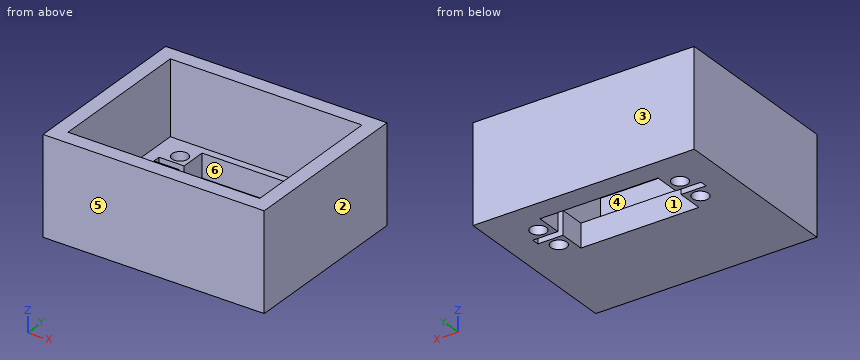
```python
from build123d import *

# Parameters (mm, degrees)
ESQUISSE1_W             = 75
ESQUISSE1_H             = 60
BOSS_EXTRU_1_DEPTH      = 8
ESQUISSE2_W             = 40
ESQUISSE2_H             = 20
ENL_V_MAT_EXTRU_1_DEPTH = 8
ESQUISSE3_W             = 8.5
ESQUISSE3_H             = 2.5
ENL_V_MAT_EXTRU_2_DEPTH = 8
ESQUISSE4_R             = 2.7
ENL_V_MAT_EXTRU_3_DEPTH = 49.685213361
ESQUISSE6_W             = 75
ESQUISSE6_H             = 60
BOSS_EXTRU_2_DEPTH      = 35
ESQUISSE7_W             = 65
ESQUISSE7_H             = 50
ENL_V_MAT_EXTRU_4_DEPTH = 35
CUT_EXTRUDE1_REACH      = 90.034
SKETCH1_W               = 10
SKETCH1_H               = 60


with BuildPart() as part:
    # Esquisse1 → Boss.-Extru.1 (new body)
    with BuildSketch(Plane.XY):
        Rectangle(ESQUISSE1_W, ESQUISSE1_H)
    extrude(amount=-BOSS_EXTRU_1_DEPTH)

    # Esquisse2 → Enlèv. mat.-Extru.1 (cut)
    with BuildSketch(Plane.XY):
        with Locations((0, 12.5)):
            Rectangle(ESQUISSE2_W, ESQUISSE2_H)
    extrude(amount=-ENL_V_MAT_EXTRU_1_DEPTH, mode=Mode.SUBTRACT)

    # Esquisse3 → Enlèv. mat.-Extru.2 (cut)
    with BuildSketch(Plane.XY):
        with Locations((-24.25, 12.5)):
            Rectangle(ESQUISSE3_W, ESQUISSE3_H)
    enl_v_mat_extru_2 = extrude(amount=-ENL_V_MAT_EXTRU_2_DEPTH, mode=Mode.SUBTRACT)

    # Esquisse4 → Enlèv. mat.-Extru.3 (cut, through all)
    with BuildSketch(Plane.XY):
        with Locations((-24, 17.5)):
            Circle(ESQUISSE4_R)
        with Locations((-24, 7.5)):
            Circle(ESQUISSE4_R)
    enl_v_mat_extru_3 = extrude(amount=-ENL_V_MAT_EXTRU_3_DEPTH, mode=Mode.SUBTRACT)

    # Symétrie2: Enlèv. mat.-Extru.2, Enlèv. mat.-Extru.3 across plane
    add(enl_v_mat_extru_2.mirror(Plane(origin=(0, 0, 0), x_dir=(0, 0, 1), z_dir=(1, 0, 0))), mode=Mode.SUBTRACT)
    add(enl_v_mat_extru_3.mirror(Plane(origin=(0, 0, 0), x_dir=(0, 0, 1), z_dir=(1, 0, 0))), mode=Mode.SUBTRACT)

    # Esquisse6 → Boss.-Extru.2 (add)
    with BuildSketch(Plane.XY):
        Rectangle(ESQUISSE6_W, ESQUISSE6_H)
    extrude(amount=BOSS_EXTRU_2_DEPTH)

    # Esquisse7 → Enlèv. mat.-Extru.4 (cut)
    with BuildSketch(Plane.XY.offset(35)):
        Rectangle(ESQUISSE7_W, ESQUISSE7_H)
    extrude(amount=-ENL_V_MAT_EXTRU_4_DEPTH, mode=Mode.SUBTRACT)

    # Cut-Extrude1: up to this face of the body (flat: up to its plane)
    cut_extrude1_end = Plane(part.part.faces().sort_by_distance((-37.5, 0, 13.5))[0])
    # Sketch1 → Cut-Extrude1 (cut, up to the picked face)
    with BuildSketch(Plane(origin=(37.5, 0, 0), x_dir=(0, 0, -1), z_dir=(1, 0, 0)), mode=Mode.PRIVATE) as cut_extrude1_sk1:
        with Locations((-30, 0)):
            Rectangle(SKETCH1_W, SKETCH1_H)
    cut_extrude1_tool1 = split(extrude(cut_extrude1_sk1.sketch, amount=-CUT_EXTRUDE1_REACH, mode=Mode.PRIVATE), bisect_by=cut_extrude1_end, keep=Keep.BOTH, mode=Mode.PRIVATE)
    add(cut_extrude1_tool1.solids().sort_by(Axis((37.5, 0, 30), (-1, 0, 0)))[0], mode=Mode.SUBTRACT)


solid = part.part
```
Part model, mm, in its own coordinate system. Face numbers are marked on the shaded views. A direction names the side the tool comes from. Round coordinates to 2 decimals unless told otherwise and drop trailing zeros. Write each loop counter-clockwise with the first axis right and the second up, starting at its lowest first coordinate (ties: lowest second). Pieces come first, ordered by that corner, then holes. Notation, with made-up numbers: M 15.25,-19.5 L 27.25,-19.5 A22 ccw 27.25,7.5 Z; hole C 79.5,-35 d8. An arc over 180 degrees is marked long. One line per question, with ' | ' between items.
(1) Probe line 1 along Y through (x, z) = (-24, -5.75); line 2 along Y through (x, z) = (-21, 23.5); line 3 along X through (y, z) = (15, 17). List the from-to ranges inside material, lowest first.
Answer key:
line 1: y = -30 to 4.8, 10.2 to 11.25, 13.75 to 14.8, 20.2 to 30 | line 2: y = -30 to -25, 25 to 30 | line 3: x = -37.5 to -32.5, 32.5 to 37.5
(2) Saw through at C-C on x = 24. Write the cut outline in (y, z).
Answer key:
outline: M -30,-8 L 4.8,-8 L 4.8,0 L -25,0 L -25,25 L -30,25 Z; M 10.2,-8 L 11.25,-8 L 11.25,0 L 10.2,0 Z; M 13.75,-8 L 14.8,-8 L 14.8,0 L 13.75,0 Z; M 20.2,-8 L 30,-8 L 30,25 L 25,25 L 25,0 L 20.2,0 Z
(3) Saw through at A-A on y = 12.5. Write the cut outline in (x, z).
Answer key:
outline: M -37.5,-8 L -28.5,-8 L -28.5,0 L -32.5,0 L -32.5,25 L -37.5,25 Z; M 28.5,-8 L 37.5,-8 L 37.5,25 L 32.5,25 L 32.5,0 L 28.5,0 Z
(4) Saw through at B-B on z = 15.5. Write the cut outline in (x, y).
Answer key:
outline: M -37.5,-30 L 37.5,-30 L 37.5,30 L -37.5,30 Z; hole M -32.5,-25 L 32.5,-25 L 32.5,25 L -32.5,25 Z
(5) Two-plate mould, pull along Y, no slides. Class the marked faces 1, 2 and 3: released by +Y, released by -Y, zero draft, split by the parting line, or undercut.
Answer key:
face 1: undercut | face 2: zero draft | face 3: released by +Y
(6) 3-axis set-ups, long thin cutter, end or side, ignore diameter. For the marked faces 4, 5 and 6: which of +Z, -Z, +X, -X, +Y, -Y reach the whole face in a straight line?
Answer key:
face 4: +Z | face 5: +Z, -Z, +X, -X, -Y | face 6: +Z, -Z
(7) Pin check, flat tips, straight feed: pin 1 (7 mm diameter, centred on x = -24, y = 7.5, fed in from +Z); pin 2 (4.5 mm diameter, centred on x = 24, y = 7.5, fed in from -Z). Stop position of each tip, or through.
Answer key:
pin 1: stops at z = 0 | pin 2: passes through
(8) Saw through at D-D on z = -5.5. Write the cut outline in (x, y), then the cut area to 3 significant figures.
Answer key:
outline: M -37.5,-30 L 37.5,-30 L 37.5,30 L -37.5,30 Z; hole M -28.5,11.25 L -20,11.25 L -20,2.5 L 20,2.5 L 20,11.25 L 28.5,11.25 L 28.5,13.75 L 20,13.75 L 20,22.5 L -20,22.5 L -20,13.75 L -28.5,13.75 Z; hole C -24,7.5 d5.4; hole C -24,17.5 d5.4; hole C 24,7.5 d5.4; hole C 24,17.5 d5.4 | area: 3,570 mm^2
